from build123d import *

# Parameters (mm, degrees)
SKETCH1_R               = 48.8061
EXTRUDE1_DEPTH          = 6.5024
CHAMFER2_SIZE           = 7.50062
CHAMFER2_SIZE2          = 9.95365893
SKETCH6_R               = 41.30548
SKETCH6_R_2             = 40.79748
EXTRUDE_THIN2_DEPTH     = 0.0254
CUT_EXTRUDE1_DEPTH      = 70.330245689
CUT_EXTRUDE1_DEPTH_BACK = 70.330245689
SKETCH7_W               = 97.6122
SKETCH7_H               = 2.9972


with BuildPart() as part:
    # Sketch1 → Extrude1 (new, symmetric)
    with BuildSketch(Plane(origin=(0, 0, 0), x_dir=(1, 0, 0), z_dir=(0, 1, 0))):
        with Locations(Location((0, 0, 0), (0, 0, 270))):
            Circle(SKETCH1_R)
    extrude(amount=EXTRUDE1_DEPTH, both=True)

    # Chamfer2
    chamfer2_edges = [part.edges().sort_by_distance(p)[0] for p in [
        (0, -6.5024, -48.8061),
    ]]
    chamfer2_side = [part.faces().sort_by_distance(p)[0] for p in [
        (0, -6.5024, 0),
    ]]
    chamfer(chamfer2_edges, length=CHAMFER2_SIZE, length2=CHAMFER2_SIZE2, reference=chamfer2_side[0])

    # Sketch6 → Extrude-Thin2 (add)
    with BuildSketch(Plane.XZ.offset(6.5024)):
        Circle(SKETCH6_R)
        Circle(SKETCH6_R_2, mode=Mode.SUBTRACT)
    extrude(amount=EXTRUDE_THIN2_DEPTH)

    # Sketch7 → Cut-Extrude1 (cut, two sides: drawn at the far end of the back side and taken through both)
    with BuildSketch(Plane(origin=(0, 0, 0), x_dir=(0, 0, -1), z_dir=(1, 0, 0)).offset(-CUT_EXTRUDE1_DEPTH_BACK)):
        with Locations((0, 5.0038)):
            Rectangle(SKETCH7_W, SKETCH7_H)
    extrude(amount=CUT_EXTRUDE1_DEPTH + CUT_EXTRUDE1_DEPTH_BACK, mode=Mode.SUBTRACT)


solid = part.part
The model under review builds one solid part; all positions refer to its coordinate system, in mm. Give positions to 0.01 mm unless a question says otherwise; leave off trailing zeros. Order: outer loops, then holes, each group sorted by start corner. A loop starts at its lowest first (then second) coordinate and runs counter-clockwise, first axis right, second up. Notation, with made-up numbers: (25.5, 14.5) -> (70.5, 14.5) arc R22 ccw to (70.5, 41.5) -> close; hole circle Ø2 at (35, 65). An arc over 180 degrees is marked (long way). Write item = value, one per line. Start each with the question number.
(1) Take a section at C-C (y = -5). Write out the cut boundary in (x, z).
(2) For pin 1 Ø4 at (x, y) = (-32, 2.5) entering from +Z; pin 2 Ø1 at (y, z) = (-4, -31.5) entering from +X; pin 3 Ø3 at (y, z) = (-4.5, 0.5) entering from +X, all flat-tipped, find the tip position at first contact; note any pin that passes through.
(3) For L1, parallel to Y at x = 23, z = 10; L2, parallel to Y at x = -29, z = 36.5; L3, parallel to Z at x = -29.5, y = -1.5, list the stretches that pass through material, from the lowest coordinate up. Write a range as from..to.
Returned:
q1.outline = circle Ø84.88 at (0, 0)
q2.pin_1 = 38.31
q2.pin_2 = 30.31
q2.pin_3 = 43.94
q3.L1 = -6.5..3.51
q3.L2 = 0.55..3.51
q3.L3 = -34.08..34.08
